Design review of the part built by this model. Coordinates are the model's own, in mm. Face numbers are marked on the shaded views. A direction names the side the tool comes from. Round coordinates to 2 decimals unless told otherwise and drop trailing zeros. Loops run counter-clockwise (first coordinate to the right, second up) from the corner with the lowest first, then second, coordinate; pieces in that order, holes last. Notation, with made-up numbers: M -25,29.5 L 22,29.5 A16 cw 22,48.5 Z; hole C -7.5,36 d8. An arc over 180 degrees is marked long. Answer as CSV lines item,"result". Start each with the question number.
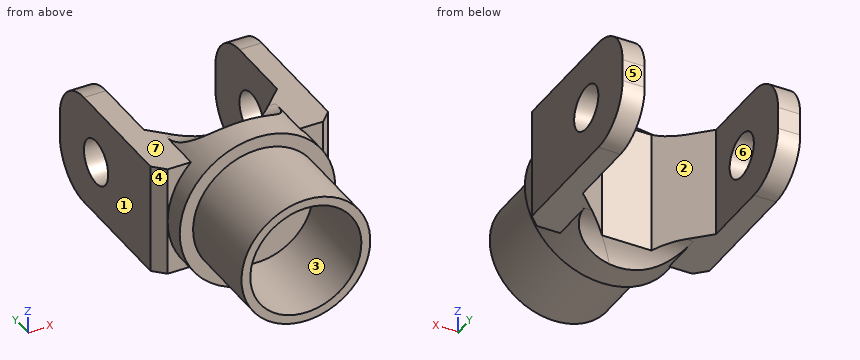
from build123d import *

# Parameters (mm, degrees)
SKETCH2_R           = 18.415
SKETCH2_R_2         = 15.875
BOSS_EXTRUDE1_DEPTH = 25.4
SKETCH3_R           = 22.225
BOSS_EXTRUDE2_DEPTH = 6.35
SKETCH5_W           = 50.8
SKETCH5_H           = 31.75
BOSS_EXTRUDE3_DEPTH = 50.8
CUT_EXTRUDE2_DEPTH  = 50.8
FILLET1_R           = 12.7
SKETCH9_R           = 6.35
CUT_EXTRUDE3_DEPTH  = 100.443919497
FILLET2_R           = 12.7


with BuildPart() as part:
    # Sketch2 → Boss-Extrude1 (new body)
    with BuildSketch(Plane(origin=(0, 0, 0), x_dir=(1, 0, 0), z_dir=(0, 1, 0))):
        with Locations(Location((0, 0, 0), (0, 0, 270))):
            Circle(SKETCH2_R)
        with Locations(Location((0, 0, 0), (0, 0, 270))):
            Circle(SKETCH2_R_2, mode=Mode.SUBTRACT)
    extrude(amount=BOSS_EXTRUDE1_DEPTH)

    # Sketch3 → Boss-Extrude2 (add)
    with BuildSketch(Plane(origin=(0, 25.4, 0), x_dir=(1, 0, 0), z_dir=(0, 1, 0))):
        with Locations(Location((0, 0, 0), (0, 0, 270))):
            Circle(SKETCH3_R)
    extrude(amount=BOSS_EXTRUDE2_DEPTH)

    # Sketch5 → Boss-Extrude3 (add)
    with BuildSketch(Plane(origin=(0, 31.75, 0), x_dir=(1, 0, 0), z_dir=(0, 1, 0))):
        Rectangle(SKETCH5_W, SKETCH5_H)
    extrude(amount=BOSS_EXTRUDE3_DEPTH)

    # Sketch7 → Cut-Extrude2 (cut)
    with BuildSketch(Plane.XY.offset(15.875)):
        Polygon((19.05, 82.55), (-19.05, 82.55), (-19.05, 50.084319149), (-7.065680851, 38.1), (7.065680851, 38.1), (19.05, 50.084319149), align=None)
        Polygon((-22.225, 31.75), (-25.4, 34.925), (-25.4, 31.75), align=None)
        Polygon((22.225, 31.75), (25.4, 34.925), (25.4, 31.75), align=None)
    extrude(amount=-CUT_EXTRUDE2_DEPTH, mode=Mode.SUBTRACT)

    # Fillet1
    fillet1_edges = [part.edges().sort_by_distance(p)[0] for p in [
        (22.225, 82.55, -15.875),
        (-22.225, 82.55, 15.875),
        (-22.225, 82.55, -15.875),
        (22.225, 82.55, 15.875),
    ]]
    fillet(fillet1_edges, radius=FILLET1_R)

    # Sketch9 → Cut-Extrude3 (cut, through all)
    with BuildSketch(Plane.ZY.offset(25.4)):
        with Locations((0, 63.5)):
            Circle(SKETCH9_R)
    extrude(amount=-CUT_EXTRUDE3_DEPTH, mode=Mode.SUBTRACT)

    # Fillet2
    # the kernel refuses this fillet: 12.7 mm, written as the material it adds along each edge
    with BuildSketch(Plane(origin=(-47.304259867, 31.75, 15.875), x_dir=(0, 1, 0), z_dir=(1, 0, 0))) as fillet2_piece_1_section:
        with BuildLine():
            CenterArc((FILLET2_R, FILLET2_R), FILLET2_R, 180, 90)
            Line((0, FILLET2_R), (0, 0))
            Line((0, 0), (FILLET2_R, 0))
        make_face()
    fillet2_piece_1 = extrude(amount=94.608519733, mode=Mode.PRIVATE)
    fillet2_piece_1 = split(fillet2_piece_1, bisect_by=Plane(origin=(-10.08116257, 41.115481719, 16.394719063), z_dir=(-0.7071067811865479, -0.7071067811865472, 0)), keep=Keep.TOP, mode=Mode.PRIVATE)
    fillet2_piece_1 = fillet2_piece_1 & Plane(origin=(0, 39.477824878, 0), x_dir=(0, 0, 1), z_dir=(0, -1, 0)) * Cylinder(22.225, 241, mode=Mode.PRIVATE)
    add(fillet2_piece_1)
    with BuildSketch(Plane(origin=(-47.304259867, 31.75, 15.875), x_dir=(0, 1, 0), z_dir=(1, 0, 0))) as fillet2_piece_2_section:
        with BuildLine():
            CenterArc((FILLET2_R, FILLET2_R), FILLET2_R, 180, 90)
            Line((0, FILLET2_R), (0, 0))
            Line((0, 0), (FILLET2_R, 0))
        make_face()
    fillet2_piece_2 = extrude(amount=94.608519733, mode=Mode.PRIVATE)
    fillet2_piece_2 = split(fillet2_piece_2, bisect_by=Plane(origin=(1e-09, 38.1, 17.97624181), z_dir=(0, -1, 0)), keep=Keep.TOP, mode=Mode.PRIVATE)
    fillet2_piece_2 = fillet2_piece_2 & Plane(origin=(0, 35.120576784, 0), x_dir=(0, 0, 1), z_dir=(0, -1, 0)) * Cylinder(22.225, 241, mode=Mode.PRIVATE)
    add(fillet2_piece_2)
    with BuildSketch(Plane(origin=(-47.304259867, 31.75, 15.875), x_dir=(0, 1, 0), z_dir=(1, 0, 0))) as fillet2_piece_3_section:
        with BuildLine():
            CenterArc((FILLET2_R, FILLET2_R), FILLET2_R, 180, 90)
            Line((0, FILLET2_R), (0, 0))
            Line((0, 0), (FILLET2_R, 0))
        make_face()
    fillet2_piece_3 = extrude(amount=94.608519733, mode=Mode.PRIVATE)
    fillet2_piece_3 = split(fillet2_piece_3, bisect_by=Plane(origin=(10.081162473, 41.115481622, 16.394719049), z_dir=(0.7071067811865472, -0.7071067811865478, 0)), keep=Keep.TOP, mode=Mode.PRIVATE)
    fillet2_piece_3 = fillet2_piece_3 & Plane(origin=(0, 39.477824822, 0), x_dir=(0, 0, 1), z_dir=(0, -1, 0)) * Cylinder(22.225, 241, mode=Mode.PRIVATE)
    add(fillet2_piece_3)
    with BuildSketch(Plane(origin=(47.304259867, 31.75, -15.875), x_dir=(0, 1, 0), z_dir=(-1, 0, 0))) as fillet2_piece_4_section:
        with BuildLine():
            CenterArc((FILLET2_R, FILLET2_R), FILLET2_R, 180, 90)
            Line((0, FILLET2_R), (0, 0))
            Line((0, 0), (FILLET2_R, 0))
        make_face()
    fillet2_piece_4 = extrude(amount=94.608519733, mode=Mode.PRIVATE)
    fillet2_piece_4 = split(fillet2_piece_4, bisect_by=Plane(origin=(10.08116257, 41.115481719, -16.394719063), z_dir=(0.7071067811865472, -0.7071067811865478, 0)), keep=Keep.TOP, mode=Mode.PRIVATE)
    fillet2_piece_4 = fillet2_piece_4 & Plane(origin=(0, 39.477824879, 0), x_dir=(0, 0, 1), z_dir=(0, -1, 0)) * Cylinder(22.225, 241, mode=Mode.PRIVATE)
    add(fillet2_piece_4)
    with BuildSketch(Plane(origin=(47.304259867, 31.75, -15.875), x_dir=(0, 1, 0), z_dir=(-1, 0, 0))) as fillet2_piece_5_section:
        with BuildLine():
            CenterArc((FILLET2_R, FILLET2_R), FILLET2_R, 180, 90)
            Line((0, FILLET2_R), (0, 0))
            Line((0, 0), (FILLET2_R, 0))
        make_face()
    fillet2_piece_5 = extrude(amount=94.608519733, mode=Mode.PRIVATE)
    fillet2_piece_5 = split(fillet2_piece_5, bisect_by=Plane(origin=(0, 38.1, -17.976241803), z_dir=(0, -1, 0)), keep=Keep.TOP, mode=Mode.PRIVATE)
    fillet2_piece_5 = fillet2_piece_5 & Plane(origin=(0, 35.120576783, 0), x_dir=(0, 0, 1), z_dir=(0, -1, 0)) * Cylinder(22.225, 241, mode=Mode.PRIVATE)
    add(fillet2_piece_5)
    with BuildSketch(Plane(origin=(47.304259867, 31.75, -15.875), x_dir=(0, 1, 0), z_dir=(-1, 0, 0))) as fillet2_piece_6_section:
        with BuildLine():
            CenterArc((FILLET2_R, FILLET2_R), FILLET2_R, 180, 90)
            Line((0, FILLET2_R), (0, 0))
            Line((0, 0), (FILLET2_R, 0))
        make_face()
    fillet2_piece_6 = extrude(amount=94.608519733, mode=Mode.PRIVATE)
    fillet2_piece_6 = split(fillet2_piece_6, bisect_by=Plane(origin=(-10.081162473, 41.115481622, -16.394719049), z_dir=(-0.7071067811865479, -0.7071067811865472, 0)), keep=Keep.TOP, mode=Mode.PRIVATE)
    fillet2_piece_6 = fillet2_piece_6 & Plane(origin=(0, 39.477824822, 0), x_dir=(0, 0, 1), z_dir=(0, -1, 0)) * Cylinder(22.225, 241, mode=Mode.PRIVATE)
    add(fillet2_piece_6)


solid = part.part
Item 1: Consider section C-C, the plane y = 39. Write out the cut boundary in (x, z) (3 decimals).
Item 2: Consider section D-D, the plane x = -5. Write out the cut boundary in (y, z) (3 decimals).
Item 3: The part is to be moulded in two halves that separate along Y. For the marked faces 4, 5, 6 and 7, say which applies: +Y half, -Y half, draft (parallel to the pull), parting line (faces both ways), or undercut.
Item 4: Consider section A-A, the plane y = 63.5. Write out the cut boundary in (x, z) (3 decimals).
Item 5: Tool access review of the marked faces 1, 2 and 3: name each direction out of +Z, -Z, +X, -X, +Y, -Y from which nothing blocks a thin tool from reaching the whole face with its end or side.
Item 6: Insertion check: pin 1 Ø16 at (y, z) = (69.5, -2) entering from -X; pin 2 Ø19 at (x, z) = (0, 0) entering from +Y; pin 3 Ø3 at (x, z) = (17.5, 6.5) entering from +Y; pin 4 Ø3.5 at (x, y) = (19, 44.5) entering from +Z (3 decimals). Each pin has a flat end and moves straight along its axis. Give the tip position at first contact, or say it passes through.
Item 7: To check wall thickness, follow line 1 (Z direction, x = 23, y = 63) (3 decimals); line 2 (X direction, y = 60, z = 14). State the ranges of each line that lie inside material, in increasing order.
Item 8: Consider section B-B, the plane z = -5. Count the separate pieces of the cut face and the enclosed holes in it, then the cut area to 3 significant figures.
Found:
1,outline,"M -25.4,-15.875 L -15.554,-15.875 A22.225 ccw -14.192,-17.104 L -7.966,-17.104 L -7.966,17.104 L -14.192,17.104 A22.225 ccw -15.554,15.875 L -25.4,15.875 Z; M 7.966,-17.104 L 14.192,-17.104 A22.225 ccw 15.554,-15.875 L 25.4,-15.875 L 25.4,15.875 L 15.554,15.875 A22.225 ccw 14.192,17.104 L 7.966,17.104 Z"
2,outline,"M 0,-17.723 L 25.4,-17.723 L 25.4,-21.655 L 33.801,-21.655 A12.7 cw 38.1,-17.576 L 38.1,17.576 A12.7 cw 33.801,21.655 L 25.4,21.655 L 25.4,17.723 L 0,17.723 L 0,15.067 L 25.4,15.067 L 25.4,-15.067 L 0,-15.067 Z"
3,face 4,"-Y half"
3,face 5,"+Y half"
3,face 6,"undercut"
3,face 7,"draft"
4,outline,"M -25.4,-15.875 L -19.05,-15.875 L -19.05,-6.35 L -25.4,-6.35 Z; M -25.4,6.35 L -19.05,6.35 L -19.05,15.875 L -25.4,15.875 Z; M 19.05,-15.875 L 25.4,-15.875 L 25.4,-6.35 L 19.05,-6.35 Z; M 19.05,6.35 L 25.4,6.35 L 25.4,15.875 L 19.05,15.875 Z"
5,face 1,"+Z, -Z, -X, +Y, -Y"
5,face 2,"+Z, -Z, +Y"
5,face 3,"-Y"
6,pin 1,"stops at x = -25.4"
6,pin 2,"stops at y = 40.53"
6,pin 3,"stops at y = 50.03"
6,pin 4,"stops at z = 15.875"
7,line 1,"z = -15.875 to -6.33, 6.33 to 15.875"
7,line 2,"x = -25.4 to -19.05, 19.05 to 25.4"
8,separate pieces,"3"
8,enclosed holes,"0"
8,area,"1,330 mm^2"
